The listing builds one solid part. Answer for the finished solid, in the listing's coordinates (mm). Give positions to 0.01 mm unless a question says otherwise; leave off trailing zeros. Write each loop counter-clockwise with the first axis right and the second up, starting at its lowest first coordinate (ties: lowest second). Pieces come first, ordered by that corner, then holes. Notation, with made-up numbers: (-33, 28.5) - (-8, 28.5) arc R20 ccw to (-8, 43.5) - close; hole circle Ø1 at (-30.5, 12). An arc over 180 degrees is marked (long way). Answer as CSV lines item,"result". Start each with the question number.
(1) Straight lines are drawn through the part: probe 1 along Z at (x, y) = (105, 0.25); probe 2 along X at (y, z) = (-0.1, 8.5); probe 3 along X at (y, z) = (-0.4, 18). For each, find the intervals that lie inside material, in ascending order.
(2) Find section A-A (y = -0.15). State how many separate pieces and enclosed holes the cut face has, then the cut area to 3 significant figures.
(3) Find section C-C (z = 35). Write down the section's boundary in (x, y).
(4) Find section B-B (x = -61.5). Write down the section's boundary in (y, z).
from build123d import *

# Parameters (mm, degrees)
SKETCH_R       = 1.65
PAD_DEPTH      = 0.75
PAD_DEPTH_BACK = 0.75


with BuildPart() as part:
    # Sketch → Pad (new body, two sides)
    with BuildSketch(Plane.XZ) as pad_sk:
        with BuildLine():
            Line((-110, -41), (-110, -31))
            ThreePointArc((-97.745166, -1.414214), (-106.815072, -14.988288), (-110, -31))
            Line((-97.745166, -1.414214), (-68.046681, 28.284271))
            ThreePointArc((-39.76241, 40), (-55.069747, 36.955181), (-68.046681, 28.284271))
            Line((-39.76241, 40), (110, 40))
            Line((110, 40), (110, -41))
            Line((110, -41), (-110, -41))
        make_face()
        with Locations((105, 30)):
            Circle(SKETCH_R, mode=Mode.SUBTRACT)
        with Locations((20, 30)):
            Circle(SKETCH_R, mode=Mode.SUBTRACT)
        with Locations((20, 10)):
            Circle(SKETCH_R, mode=Mode.SUBTRACT)
        with Locations((105, 10)):
            Circle(SKETCH_R, mode=Mode.SUBTRACT)
        with Locations((105, -30)):
            Circle(SKETCH_R, mode=Mode.SUBTRACT)
        with Locations((20, -30)):
            Circle(SKETCH_R, mode=Mode.SUBTRACT)
        with Locations((20, -10)):
            Circle(SKETCH_R, mode=Mode.SUBTRACT)
        with Locations((105, -10)):
            Circle(SKETCH_R, mode=Mode.SUBTRACT)
    extrude(amount=PAD_DEPTH)
    extrude(pad_sk.sketch, amount=-PAD_DEPTH_BACK)


solid = part.part
Result set:
1,probe 1,"-41 to -31.65, -28.35 to -11.65, -8.35 to 8.35, 11.65 to 28.35, 31.65 to 40"
1,probe 2,"-87.83 to 19.31, 20.69 to 104.31, 105.69 to 110"
1,probe 3,"-78.33 to 110"
2,separate pieces,"1"
2,enclosed holes,"8"
2,area,"16,200 mm^2"
3,outline,"(-59.13, -0.75) - (110, -0.75) - (110, 0.75) - (-59.13, 0.75) - close"
4,outline,"(-0.75, -41) - (0.75, -41) - (0.75, 33.58) - (-0.75, 33.58) - close"
